For this review, take the finished solid that the model builds, in its own axes (mm). A direction names the side the tool comes from. Coordinates: 2 decimals unless noted, no trailing zeros. Order: outer loops, then holes, each group sorted by start corner. A loop starts at its lowest first (then second) coordinate and runs counter-clockwise, first axis right, second up. Notation, with made-up numbers: (-30, -18) -> (-22, -18) arc R20 ccw to (-22, -14) -> close; hole circle Ø1 at (71.5, -40). An arc over 180 degrees is marked (long way). Answer as a JSON object with one key per item and string values. Group by question number.
1) Draft analysis for pull direction Y (two halves, no side actions). For faces 4 (the flat face through (142.75, 50, 2)), 5 (the flat face through (76, 150, -7)), 6 (the flat face through (74, 0, 2)), state which applies: +Y half, -Y half, draft (parallel to the pull), parting line (faces both ways), or undercut.
2) Wall thickness on L1, parallel to X at y = 102, z = 2.95; L2, parallel to X at y = 73.5, z = 1.65; L3, parallel to Y at x = 13, z = 1.3: over which ranges is each line inside the solid? List them lowest first.
3) Add section A-A, the plane x = 140. Write out the cut boundary in (y, z), then the cut area to 3 significant figures.
4) Add section B-B, the plane x = 105.5. Write out the cut boundary in (y, z).
5) Machinability: for faces 1 (the flat face through (76, 148, -18)), 2 (the flat face through (76, 146, -9)), 3 (the cylindrical face through (140.06, 107.25, 1.97)), which of the approach directions +Z, -Z, +X, -X, +Y, -Y give a long, thin tool a straight path to every point of the face, cutting with its end or side? Answer none if there is none.
6) Add section C-C, the plane z = -4.5. Write out the cut boundary in (x, y).
7) Add section D-D, the plane y = 96. Write out the cut boundary in (x, z).
8) For pin 1 (3.5 mm diameter, centred on x = 95, y = 45, fed in from -Z); pin 2 (2 mm diameter, centred on x = 133, z = -11, fed in from -Y), all flat-tipped, find the tip position at first contact; note any pin that passes through.
from build123d import *

# Parameters (mm, degrees)
SKETCH_1_W      = 150
SKETCH_1_H      = 150
SKETCH_1_R      = 1.5
EXTRUDE_1_DEPTH = 4
SKETCH_2_W      = 150
SKETCH_2_H      = 4
EXTRUDE_2_DEPTH = 18


with BuildPart() as part:
    # 草图1 → 凸台-拉伸1 (new body)
    with BuildSketch(Plane.XY):
        with Locations((75, 75)):
            Rectangle(SKETCH_1_W, SKETCH_1_H)
        with Locations((95, 102)):
            Circle(SKETCH_1_R, mode=Mode.SUBTRACT)
        with Locations((95, 45)):
            Circle(SKETCH_1_R, mode=Mode.SUBTRACT)
        with Locations((95, 73.5)):
            Circle(SKETCH_1_R, mode=Mode.SUBTRACT)
        with Locations((13, 102)):
            Circle(SKETCH_1_R, mode=Mode.SUBTRACT)
        with BuildLine():
            Line((142.75, 130), (142.75, 110))
            ThreePointArc((142.75, 110), (140, 107.25), (137.25, 110))
            Line((137.25, 110), (137.25, 130))
            ThreePointArc((137.25, 130), (140, 132.75), (142.75, 130))
        make_face(mode=Mode.SUBTRACT)
        with BuildLine():
            Line((142.75, 60), (142.75, 40))
            ThreePointArc((142.75, 40), (140, 37.25), (137.25, 40))
            Line((137.25, 40), (137.25, 60))
            ThreePointArc((137.25, 60), (140, 62.75), (142.75, 60))
        make_face(mode=Mode.SUBTRACT)
    extrude(amount=EXTRUDE_1_DEPTH)

    # 草图2 → 凸台-拉伸2 (add)
    with BuildSketch(Plane(origin=(0, 0, 0), x_dir=(-1, 0, 0), z_dir=(0, 0, -1))):
        with Locations((-75, 148)):
            Rectangle(SKETCH_2_W, SKETCH_2_H)
    extrude(amount=EXTRUDE_2_DEPTH)


solid = part.part
Output values:
{
 "1": {"face 4": "undercut", "face 5": "+Y half", "face 6": "-Y half"},
 "2": {"L1": "x = 0 to 11.5, 14.5 to 93.5, 96.5 to 150", "L2": "x = 0 to 93.5, 96.5 to 150", "L3": "y = 0 to 100.5, 103.5 to 150"},
 "3": {"outline": "(0, 0) -> (37.25, 0) -> (37.25, 4) -> (0, 4) -> close; (62.75, 0) -> (107.25, 0) -> (107.25, 4) -> (62.75, 4) -> close; (132.75, 0) -> (146, 0) -> (146, -18) -> (150, -18) -> (150, 4) -> (132.75, 4) -> close", "area": "468 mm²"},
 "4": {"outline": "(0, 0) -> (146, 0) -> (146, -18) -> (150, -18) -> (150, 4) -> (0, 4) -> close"},
 "5": {"face 1": "-Z, +X, -X, +Y, -Y", "face 2": "-Z, +X, -X, -Y", "face 3": "+Z, -Z"},
 "6": {"outline": "(0, 146) -> (150, 146) -> (150, 150) -> (0, 150) -> close"},
 "7": {"outline": "(0, 0) -> (150, 0) -> (150, 4) -> (0, 4) -> close"},
 "8": {"pin 1": "stops at z = 0", "pin 2": "stops at y = 146"}
}
